Work out the finished part from the listing and answer in its coordinate system (mm). A direction names the side the tool comes from. Round coordinates to 2 decimals unless told otherwise and drop trailing zeros. Order: outer loops, then holes, each group sorted by start corner. A loop starts at its lowest first (then second) coordinate and runs counter-clockwise, first axis right, second up. Notation, with made-up numbers: (-31, -17) - (-27, -17) arc R19 ccw to (-27, -9) - close; hole circle Ø7 at (79, 86). An arc over 180 degrees is marked (long way). Answer in a Markdown table with one row per item.
from build123d import *

# Parameters (mm, degrees)
BOSS_EXTRUDE1_DEPTH = 5
SKETCH3_W           = 41.9
SKETCH3_H           = 20
CUT_EXTRUDE1_DEPTH  = 135.489776563


with BuildPart() as part:
    # Sketch2 → Boss-Extrude1 (new body)
    with BuildSketch(Plane(origin=(0, 0, 0), x_dir=(1, 0, 0), z_dir=(0, 1, 0))):
        with BuildLine():
            Line((24.109126902, 15), (85.890873098, 15))
            ThreePointArc((85.890873098, 15), (91.831758355, 15.902725787), (97.236344581, 18.529411765))
            ThreePointArc((97.236344581, 18.529411765), (132.5, 0), (97.236344581, -18.529411765))
            ThreePointArc((97.236344581, -18.529411765), (91.831758355, -15.902725787), (85.890873098, -15))
            Line((85.890873098, -15), (24.109126902, -15))
            ThreePointArc((24.109126902, -15), (18.168241645, -15.902725787), (12.763655419, -18.529411765))
            ThreePointArc((12.763655419, -18.529411765), (-22.5, 0), (12.763655419, 18.529411765))
            ThreePointArc((12.763655419, 18.529411765), (18.168241645, 15.902725787), (24.109126902, 15))
        make_face()
    extrude(amount=BOSS_EXTRUDE1_DEPTH)

    # Sketch3 → Cut-Extrude1 (cut, through all)
    with BuildSketch(Plane(origin=(0, 5, 0), x_dir=(1, 0, 0), z_dir=(0, 1, 0))):
        with Locations((100, 0)):
            Rectangle(SKETCH3_W, SKETCH3_H)
    extrude(amount=-CUT_EXTRUDE1_DEPTH, mode=Mode.SUBTRACT)


solid = part.part
1) Find section B-B, the plane z = 0. Give the vertices of the cut face in (x, y).
Filled in:
| item | result |
|---|---|
| outline | (-22.5, 0) - (79.05, 0) - (79.05, 5) - (-22.5, 5) - close; (120.95, 0) - (132.5, 0) - (132.5, 5) - (120.95, 5) - close |
2) Find section C-C, the plane y = 4.1. Give the vertices of the cut face in (x, z), then the cut area to 3 significant figures.
Filled in:
| item | result |
|---|---|
| outline | (12.76, -18.53) arc R20 cw to (24.11, -15) - (85.89, -15) arc R20 cw to (97.24, -18.53) arc R22.5 ccw (long way) to (97.24, 18.53) arc R20 cw to (85.89, 15) - (24.11, 15) arc R20 cw to (12.76, 18.53) arc R22.5 ccw (long way) to start; hole (79.05, -10) - (120.95, -10) - (120.95, 10) - (79.05, 10) - close |
| area | 4,420 mm^2 |
3) Which of the six approach directions +Z, -Z, +X, -X, +Y, -Y give full straight-line access (tool end or side, diameter ignored) to faces 1 (the face through (18.249, 2.465, 15.878)), 2 (the face through (18.088, 2.465, -15.928)), 3 (the face through (100, 3, -10))?
Filled in:
| item | result |
|---|---|
| face 1 | +Z, +Y, -Y |
| face 2 | -Z, +Y, -Y |
| face 3 | +Y, -Y |
4) Find section A-A, the plane x = 110. Give the vertices of the cut face in (y, z).
Filled in:
| item | result |
|---|---|
| outline | (0, -22.5) - (5, -22.5) - (5, -10) - (0, -10) - close; (0, 10) - (5, 10) - (5, 22.5) - (0, 22.5) - close |
5) The mould has two halves that part along Z. Classify faces 4 (the face through (-22.49, 2.46, 0.68)), 5 (the face through (100, 3, 10)), 6 (the face through (55, 2, -15)): released by +Z, released by -Z, zero draft, split by the parting line, or undercut.
Filled in:
| item | result |
|---|---|
| face 4 | split by the parting line |
| face 5 | undercut |
| face 6 | released by -Z |
6) Find section D-D, the plane x = 75. Give the vertices of the cut face in (y, z), then the cut area to 3 significant figures.
Filled in:
| item | result |
|---|---|
| outline | (0, -15) - (5, -15) - (5, 15) - (0, 15) - close |
| area | 150 mm^2 |
7) Each of these flat-tipped pins is pushed along its axis until it touches: pin 1 (1.5 mm diameter, centred on y = 3, z = 2.5, fed in from -X); pin 2 (2.5 mm diameter, centred on x = 58.5, y = 1.5, fed in from +Z); pin 3 (2.5 mm diameter, centred on x = 95.5, y = 2.5, fed in from +Z). Where does it stop, or does it pass through?
Filled in:
| item | result |
|---|---|
| pin 1 | stops at x = -22.43 |
| pin 2 | stops at z = 15 |
| pin 3 | stops at z = 18.2 |
8) Find the intervals of material crossed by probe 1 along Z at (x, y) = (86, 3.7); probe 2 along Z at (x, y) = (66.5, 2.8); probe 3 along X at (y, z) = (1.9, -2), in increasing order. Write a range as from..to.
Filled in:
| item | result |
|---|---|
| probe 1 | z = -15..-10, 10..15 |
| probe 2 | z = -15..15 |
| probe 3 | x = -22.41..79.05, 120.95..132.41 |
